For this review, take the finished solid that the model builds, in its own axes (mm). Coordinates: 2 decimals unless noted, no trailing zeros. Loops run counter-clockwise (first coordinate to the right, second up) from the corner with the lowest first, then second, coordinate; pieces in that order, holes last. Notation, with made-up numbers: (12, 13) -> (43, 13) arc R16 cw to (43, 32) -> close; hole circle Ø11 at (-26, 7.25). An arc over 180 degrees is marked (long way). Answer in a Markdown table with one row per item.
from build123d import *

# Parameters (mm, degrees)
SKETCH1_R           = 75
SKETCH1_R_2         = 2.5
BOSS_EXTRUDE1_DEPTH = 6.35


with BuildPart() as part:
    # Sketch1 → Boss-Extrude1 (new body)
    with BuildSketch(Plane.XY):
        Circle(SKETCH1_R)
        with Locations((0, 30)):
            Circle(SKETCH1_R_2, mode=Mode.SUBTRACT)
        with Locations((0, 40)):
            Circle(SKETCH1_R_2, mode=Mode.SUBTRACT)
        with Locations((0, 50)):
            Circle(SKETCH1_R_2, mode=Mode.SUBTRACT)
        with Locations((0, 60)):
            Circle(SKETCH1_R_2, mode=Mode.SUBTRACT)
        with Locations((0, 70)):
            Circle(SKETCH1_R_2, mode=Mode.SUBTRACT)
        Circle(SKETCH1_R_2, mode=Mode.SUBTRACT)
    extrude(amount=BOSS_EXTRUDE1_DEPTH)


solid = part.part
Item 1: Take a section at C-C, the plane x = 0. State the section outline as (y, z) points, and give its area (3 significant figures).
Worked answers:
| item | result |
|---|---|
| outline | (-75, 0) -> (-2.5, 0) -> (-2.5, 6.35) -> (-75, 6.35) -> close; (2.5, 0) -> (27.5, 0) -> (27.5, 6.35) -> (2.5, 6.35) -> close; (32.5, 0) -> (37.5, 0) -> (37.5, 6.35) -> (32.5, 6.35) -> close; (42.5, 0) -> (47.5, 0) -> (47.5, 6.35) -> (42.5, 6.35) -> close; (52.5, 0) -> (57.5, 0) -> (57.5, 6.35) -> (52.5, 6.35) -> close; (62.5, 0) -> (67.5, 0) -> (67.5, 6.35) -> (62.5, 6.35) -> close; (72.5, 0) -> (75, 0) -> (75, 6.35) -> (72.5, 6.35) -> close |
| area | 762 mm² |
Item 2: The part is to be moulded in two halves that separate along Y. For faces 1 (the cylindrical face through (-0.54, -2.44, 3.13)), 2 (the flat face through (-1, -16, 6.35)), 3 (the cylindrical face through (-9.764, 74.362, 3.131)), say which applies: +Y half, -Y half, draft (parallel to the pull), parting line (faces both ways), or undercut.
Worked answers:
| item | result |
|---|---|
| face 1 | undercut |
| face 2 | draft |
| face 3 | parting line |
Item 3: Insertion check: pin 1 (1 mm diameter, centred on x = 48.5, z = 4.5, fed in from +Y); pin 2 (8 mm diameter, centred on x = 0, y = 0, fed in from +Z); pin 3 (3 mm diameter, centred on x = 0, y = 40, fed in from -Z); pin 4 (3 mm diameter, centred on y = 48.5, z = 3.5, fed in from -X). Each pin has a flat end and moves straight along its axis. Give the tip position at first contact, or say it passes through.
Worked answers:
| item | result |
|---|---|
| pin 1 | y = 57.63 |
| pin 2 | z = 6.35 |
| pin 3 | through |
| pin 4 | x = -58.45 |
Item 4: For L1, parallel to Y at x = -40, z = 3.5; L2, parallel to Y at x = 45, z = 6; L3, parallel to X at y = 47, z = 6, list the stretches that pass through material, from the lowest coordinate up.
Worked answers:
| item | result |
|---|---|
| L1 | -63.44 to 63.44 |
| L2 | -60 to 60 |
| L3 | -58.45 to 58.45 |
Item 5: Take a section at B-B, the plane z = 3.25. State the section outline as (x, y) points, and give its area (3 significant figures).
Worked answers:
| item | result |
|---|---|
| outline | circle Ø150 at (0, 0); hole circle Ø5 at (0, 0); hole circle Ø5 at (0, 30); hole circle Ø5 at (0, 40); hole circle Ø5 at (0, 50); hole circle Ø5 at (0, 60); hole circle Ø5 at (0, 70) |
| area | 17,600 mm² |
Item 6: Take a section at D-D, the plane y = 40. State the section outline as (x, z) points, and give its area (3 significant figures).
Worked answers:
| item | result |
|---|---|
| outline | (-63.44, 0) -> (-2.5, 0) -> (-2.5, 6.35) -> (-63.44, 6.35) -> close; (2.5, 0) -> (63.44, 0) -> (63.44, 6.35) -> (2.5, 6.35) -> close |
| area | 774 mm² |
Item 7: Take a section at A-A, the plane y = 60. State the section outline as (x, z) points.
Worked answers:
| item | result |
|---|---|
| outline | (-45, 0) -> (-2.5, 0) -> (-2.5, 6.35) -> (-45, 6.35) -> close; (2.5, 0) -> (45, 0) -> (45, 6.35) -> (2.5, 6.35) -> close |
